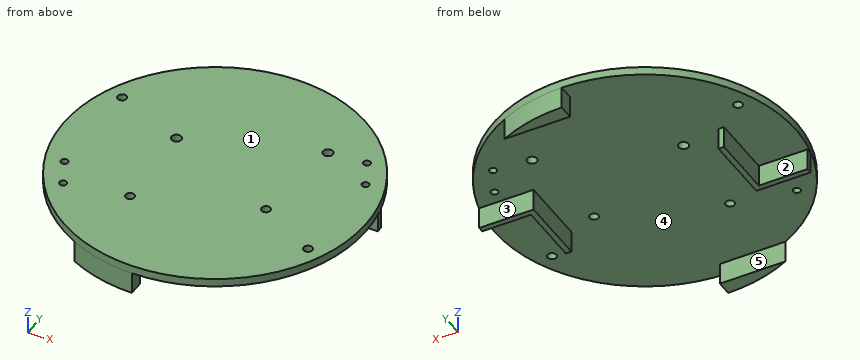
```python
from build123d import *

# Parameters (mm, degrees)
SKETCH_R        = 55
PAD_DEPTH       = 3
SKETCH003_R     = 1.3
SKETCH003_R_2   = 1.8
SKETCH003_R_3   = 1.6
POCKET_DEPTH    = 5
PAD001_DEPTH    = 11
PAD002_DEPTH    = 11
SKETCH004_R     = 1.6
POCKET001_DEPTH = 5


with BuildPart() as part:
    # Sketch → Pad (new body)
    with BuildSketch(Plane.XY):
        Circle(SKETCH_R)
    extrude(amount=PAD_DEPTH)

    # Sketch003 → Pocket (cut)
    with BuildSketch(Plane.XY.offset(3)):
        with Locations((-45, -18)):
            Circle(SKETCH003_R)
        with Locations((45, 18)):
            Circle(SKETCH003_R)
        with Locations((-40, -28)):
            Circle(SKETCH003_R)
        with Locations((40, 28)):
            Circle(SKETCH003_R)
        with Locations((-19.567712, 9.90478)):
            Circle(SKETCH003_R_2)
        with Locations((26.477227, 26.663767)):
            Circle(SKETCH003_R_2)
        with Locations((-18.019993, -23.585586)):
            Circle(SKETCH003_R_3)
        with Locations((23.326482, -8.536699)):
            Circle(SKETCH003_R_3)
    extrude(amount=-POCKET_DEPTH, mode=Mode.SUBTRACT)

    # Sketch001 (on Face3 of Pad) → Pad001 (join)
    with BuildSketch(Plane.XY.offset(3)):
        Polygon((33.500008, 0), (33.500008, 13), (53.345406, 13), (53.345406, 11), (35.5, 11), (35.5, -0.005684), (35.5, -12), (33.500008, -12), align=None)
        Polygon((-33.5, 0), (-33.5, -13), (-53.293575, -13), (-53.293575, -11), (-35.5, -11), (-35.5, 0.001212), (-35.5, 12), (-33.5, 12), align=None)
    extrude(amount=-PAD001_DEPTH)

    # Sketch002 → Pad002 (join)
    with BuildSketch(Plane.XY.offset(3)):
        with BuildLine():
            ThreePointArc((-23.973944, -49.5), (-12.298374, -53.607369), (0, -55))
            Line((0, -49.5), (0, -55))
            Line((-23.973944, -49.5), (0, -49.5))
        make_face()
        with BuildLine():
            ThreePointArc((23.973944, 49.5), (12.298374, 53.607369), (0, 55))
            Line((0, 49.5), (0, 55))
            Line((23.973944, 49.5), (0, 49.5))
        make_face()
    extrude(amount=-PAD002_DEPTH)

    # Sketch004 (on Face4 of Pad002) → Pocket001 (cut)
    with BuildSketch(Plane.XY.offset(3)):
        with Locations((-45, 20)):
            Circle(SKETCH004_R)
        with Locations((45, -20)):
            Circle(SKETCH004_R)
    extrude(amount=-POCKET001_DEPTH, mode=Mode.SUBTRACT)


solid = part.part
```
Input: part model. Units: mm. Frame: model coordinates. Face numbers are marked on the shaded views. A direction names the side the tool comes from. Give positions to 0.01 mm unless a question says otherwise; leave off trailing zeros. Order: outer loops, then holes, each group sorted by start corner. A loop starts at its lowest first (then second) coordinate and runs counter-clockwise, first axis right, second up. Notation, with made-up numbers: (78, 82) - (97, 82) arc R22 ccw to (97, 118) - close; hole circle Ø10 at (67, 72.5). An arc over 180 degrees is marked (long way). Put each result on its own line as item: value.
Item 1: Section query A-A, the plane z = -5.25. Return loops of the section in (x, y), then the cut area to 3 significant figures.
Found:
outline: (-53.29, -13) - (-33.5, -13) - (-33.5, 12) - (-35.5, 12) - (-35.5, -11) - (-53.29, -11) - close; (-23.97, -49.5) arc R55 ccw to (0, -55) - (0, -49.5) - close; (0, 49.5) - (23.97, 49.5) arc R55 ccw to (0, 55) - close; (33.5, -12) - (35.5, -12) - (35.5, 11) - (53.35, 11) - (53.35, 13) - (33.5, 13) - close
area: 349 mm^2
Item 2: Draft query along X for the marked faces 4 and 5. Return one class per face: +X half, -X half, draft (parallel to the pull), parting line (faces both ways), or undercut.
Found:
face 4: undercut
face 5: draft
Item 3: Access query for the marked faces 1, 2 and 3. Directions: +Z, -Z, +X, -X, +Y, -Y. A direction counts if a zero-diameter tool reaches every point of the face in a straight line with its end or side. Return the directions, or none.
Found:
face 1: +Z, +X, -X, +Y, -Y
face 2: -Z, -X, +Y
face 3: -Z, +X, -X, +Y
Item 4: Section query C-C, the plane x = -40. Return loops of the section in (y, z).
Found:
outline: (-37.75, 0) - (-29.3, 0) - (-29.3, 3) - (-37.75, 3) - close; (-26.7, 0) - (-13, 0) - (-13, -8) - (-11, -8) - (-11, 0) - (37.75, 0) - (37.75, 3) - (-26.7, 3) - close
Item 5: Contact query for flat-ended pins moving along their axis: pin 1 (2 mm diameter, centred on x = 34, z = -5, fed in from -Y); pin 2 (6.5 mm diameter, centred on x = -8, z = -2, fed in from +Y); pin 3 (12 mm diameter, centred on x = -1, y = 3.5, fed in from -Z); pin 4 (3 mm diameter, centred on x = -40, y = -28, fed in from +Z). Output: stop coordinate, or through.
Found:
pin 1: stops at y = -12
pin 2: stops at y = 54.73
pin 3: stops at z = 0
pin 4: stops at z = 3
Item 6: Section query B-B, the plane y = -28. Return loops of the section in (x, z), then the cut area to 3 significant figures.
Found:
outline: (-47.34, 0) - (-41.3, 0) - (-41.3, 3) - (-47.34, 3) - close; (-38.7, 0) - (47.34, 0) - (47.34, 3) - (-38.7, 3) - close
area: 276 mm^2
Item 7: Section query D-D, the plane x = 45. Return loops of the section in (y, z), then the cut area to 3 significant figures.
Found:
outline: (-31.62, 0) - (-21.6, 0) - (-21.6, 3) - (-31.62, 3) - close; (-18.4, 0) - (11, 0) - (11, -8) - (13, -8) - (13, 0) - (16.7, 0) - (16.7, 3) - (-18.4, 3) - close; (19.3, 0) - (31.62, 0) - (31.62, 3) - (19.3, 3) - close
area: 188 mm^2
Item 8: Ray query, L1, parallel to X at y = -6.5, z = -2; L2, parallel to Y at x = -40, z = 2.3; L3, parallel to Y at x = 42, z = -2. Return the intervals inside material, ascending. Write a range as from..to.
Found:
L1: x = -35.5..-33.5, 33.5..35.5
L2: y = -37.75..-29.3, -26.7..37.75
L3: y = 11..13
